Geometry check sheet. Reference: the model listing, model coordinates, mm. Face numbers are marked on the shaded views. A direction names the side the tool comes from. Round coordinates to 2 decimals unless told otherwise and drop trailing zeros. Write each loop counter-clockwise with the first axis right and the second up, starting at its lowest first coordinate (ties: lowest second). Pieces come first, ordered by that corner, then holes. Notation, with made-up numbers: (-37.75, 17) - (-32.75, 17) arc R16 ccw to (-32.75, 41) - close; hole circle Ø2 at (-12.5, -36.5). An arc over 180 degrees is marked (long way). Return JSON: item names as keys, results as strings. Group by question number.
from build123d import *

# Parameters (mm, degrees)
BOSS_EXTRU_1_DEPTH      = 1
ESQUISSE2_R             = 0.5
ENL_V_MAT_EXTRU_1_DEPTH = 10
ENL_V_MAT_EXTRU_2_DEPTH = 0.01
ENL_V_START             = -1
ENL_V_MAT_EXTRU_3_DEPTH = 0.01
BOSS_EXTRU_2_DEPTH      = 1.5
BOSS_EXTRU_2_DEPTH_BACK = 5.1
ESQUISSE5_R             = 2.275332805
BOSS_EXTRU_3_DEPTH      = 3.2
ENL_V_START_2           = -0.6
ESQUISSE6_R             = 2.275332805
ESQUISSE6_R_2           = 1.7
ENL_V_MAT_EXTRU_4_DEPTH = 2
ESQUISSE7_W             = 1.97090018
ESQUISSE7_H             = 3.898474417
ESQUISSE7_W_2           = 0.989857895
ESQUISSE7_H_2           = 1.612554693
ESQUISSE7_W_3           = 1.027355852
ESQUISSE7_W_4           = 1.146705559
ESQUISSE7_H_3           = 1.806710228
BOSS_EXTRU_4_DEPTH      = 1.5
ESQUISSE8_W             = 1.25807389
ESQUISSE8_H             = 0.666039119
ESQUISSE8_W_2           = 0.69364074
ESQUISSE8_H_2           = 1.255273727
BOSS_EXTRU_5_DEPTH      = 0.5
ESQUISSE9_W             = 3.84822602
ESQUISSE9_H             = 0.777045638
ENL_V_MAT_EXTRU_5_DEPTH = 1
CHANFREIN1_SIZE         = 0.4
ESQUISSE10_W            = 3.228737269
ESQUISSE10_H            = 1.612554693
ENL_V_MAT_EXTRU_6_DEPTH = 0.75
ESQUISSE11_W            = 1.213675147
ESQUISSE11_H            = 1.927537991
ENL_V_MAT_EXTRU_7_DEPTH = 0.5
ESQUISSE12_W            = 1.97090018
ESQUISSE12_H            = 3.898474417
BOSS_EXTRU_6_DEPTH      = 0.25
CHANFREIN2_SIZE         = 0.2
ENL_V_MAT_EXTRU_8_DEPTH = 6.25


with BuildPart() as part:
    # Esquisse1 → Boss.-Extru.1 (new body)
    with BuildSketch(Plane.XY):
        with BuildLine():
            Line((0, 11.3), (0.8, 12.1))
            Line((0.8, 12.1), (12.9, 12.1))
            ThreePointArc((12.9, 12.1), (13.5, 11.5), (14.1, 12.1))
            Line((14.1, 12.1), (15.2, 12.1))
            Line((15.2, 12.1), (16, 11.3))
            Line((16, 11.3), (16, 0.8))
            Line((16, 0.8), (15.2, 0))
            Line((15.2, 0), (14.1, 0))
            ThreePointArc((14.1, 0), (13.5, 0.6), (12.9, 0))
            Line((12.9, 0), (0.8, 0))
            Line((0.8, 0), (0, 0.8))
            Line((0, 0.8), (0, 11.3))
        make_face()
    extrude(amount=BOSS_EXTRU_1_DEPTH)

    # Esquisse2 → Enl_v. mat.-Extru.1 (cut)
    with BuildSketch(Plane.XY.offset(1)):
        with Locations((0.85, 10.25)):
            Circle(ESQUISSE2_R)
        with Locations((0.85, 1.85)):
            Circle(ESQUISSE2_R)
    extrude(amount=-ENL_V_MAT_EXTRU_1_DEPTH, mode=Mode.SUBTRACT)

    # Esquisse3 → Enl_v. mat.-Extru.2 (cut)
    with BuildSketch(Plane.XY.offset(1)):
        with BuildLine():
            Line((1.5, 9.2), (0.2, 9.2))
            ThreePointArc((0.2, 9.2), (0.058578644, 9.258578644), (0, 9.4))
            Line((0, 9.4), (0, 11.1))
            ThreePointArc((0, 11.1), (0.058578644, 11.241421356), (0.2, 11.3))
            Line((0.2, 11.3), (1.5, 11.3))
            ThreePointArc((1.5, 11.3), (1.641421356, 11.241421356), (1.7, 11.1))
            Line((1.7, 11.1), (1.7, 9.4))
            ThreePointArc((1.7, 9.4), (1.641421356, 9.258578644), (1.5, 9.2))
        make_face()
        with BuildLine():
            Line((1.5, 2.9), (0.2, 2.9))
            ThreePointArc((0.2, 2.9), (0.058578644, 2.841421356), (0, 2.7))
            Line((0, 2.7), (0, 1))
            ThreePointArc((0, 1), (0.058578644, 0.858578644), (0.2, 0.8))
            Line((0.2, 0.8), (1.5, 0.8))
            ThreePointArc((1.5, 0.8), (1.641421356, 0.858578644), (1.7, 1))
            Line((1.7, 1), (1.7, 2.7))
            ThreePointArc((1.7, 2.7), (1.641421356, 2.841421356), (1.5, 2.9))
        make_face()
    extrude(amount=-ENL_V_MAT_EXTRU_2_DEPTH, mode=Mode.SUBTRACT)

    # Esquisse3_2 → Enl_v. mat.-Extru.3 (cut)
    with BuildSketch(Plane.XY.offset(1).offset(ENL_V_START)):
        with BuildLine():
            Line((1.5, 9.2), (0.2, 9.2))
            ThreePointArc((0.2, 9.2), (0.058578644, 9.258578644), (0, 9.4))
            Line((0, 9.4), (0, 11.1))
            ThreePointArc((0, 11.1), (0.058578644, 11.241421356), (0.2, 11.3))
            Line((0.2, 11.3), (1.5, 11.3))
            ThreePointArc((1.5, 11.3), (1.641421356, 11.241421356), (1.7, 11.1))
            Line((1.7, 11.1), (1.7, 9.4))
            ThreePointArc((1.7, 9.4), (1.641421356, 9.258578644), (1.5, 9.2))
        make_face()
        with BuildLine():
            Line((1.5, 2.9), (0.2, 2.9))
            ThreePointArc((0.2, 2.9), (0.058578644, 2.841421356), (0, 2.7))
            Line((0, 2.7), (0, 1))
            ThreePointArc((0, 1), (0.058578644, 0.858578644), (0.2, 0.8))
            Line((0.2, 0.8), (1.5, 0.8))
            ThreePointArc((1.5, 0.8), (1.641421356, 0.858578644), (1.7, 1))
            Line((1.7, 1), (1.7, 2.7))
            ThreePointArc((1.7, 2.7), (1.641421356, 2.841421356), (1.5, 2.9))
        make_face()
    extrude(amount=ENL_V_MAT_EXTRU_3_DEPTH, mode=Mode.SUBTRACT)

    # Esquisse4 → Boss.-Extru.2 (add, two sides)
    with BuildSketch(Plane(origin=(16, 0, 0), x_dir=(0, 0, -1), z_dir=(1, 0, 0))) as boss_extru_2_sk:
        with BuildLine():
            Line((-4.2, 3.2), (-4.2, 8.9))
            ThreePointArc((-4.2, 8.9), (-2.6, 10.5), (-1, 8.9))
            Line((-1, 8.9), (-1, 3.2))
            ThreePointArc((-1, 3.2), (-2.6, 1.6), (-4.2, 3.2))
        make_face()
    extrude(amount=BOSS_EXTRU_2_DEPTH)
    extrude(boss_extru_2_sk.sketch, amount=-BOSS_EXTRU_2_DEPTH_BACK)

    # Esquisse5 → Boss.-Extru.3 (add)
    with BuildSketch(Plane.XY.offset(1)):
        with Locations((4.830231602, 2.627298973)):
            Circle(ESQUISSE5_R)
    extrude(amount=BOSS_EXTRU_3_DEPTH)

    # Esquisse6 → Enl_v. mat.-Extru.4 (cut)
    with BuildSketch(Plane.XY.offset(4.2).offset(ENL_V_START_2)):
        with Locations((4.830231602, 2.627298973)):
            Circle(ESQUISSE6_R)
        with Locations((4.830231602, 2.627298973)):
            Circle(ESQUISSE6_R_2, mode=Mode.SUBTRACT)
    extrude(amount=-ENL_V_MAT_EXTRU_4_DEPTH, mode=Mode.SUBTRACT)

    # Esquisse7 → Boss.-Extru.4 (add)
    with BuildSketch(Plane.XY.offset(1)):
        Polygon((4.12719031, 7.97411301), (4.460209869, 7.97411301), (4.460209869, 8.751158648), (5.200253335, 8.751158648), (5.200253335, 7.97411301), (5.644279414, 7.97411301), (5.644279414, 8.751158648), (6.310318533, 8.751158648), (6.310318533, 7.97411301), (6.754344612, 7.97411301), (6.754344612, 6.087002173), (6.310318533, 6.087002173), (6.310318533, 5.309956535), (5.644279414, 5.309956535), (5.644279414, 6.087002173), (5.200253335, 6.087002173), (5.200253335, 5.309956535), (4.460209869, 5.309956535), (4.460209869, 6.087002173), (4.12719031, 6.087002173), (4.12719031, 5.309956535), (3.387146845, 5.309956535), (3.387146845, 6.087002173), (2.906118592, 6.087002173), (2.906118592, 7.97411301), (3.387146845, 7.97411301), (3.387146845, 8.751158648), (4.12719031, 8.751158648), align=None)
        with Locations((8.659747019, 7.97411301)):
            Rectangle(ESQUISSE7_W, ESQUISSE7_H)
        with Locations((3.757168577, 10.711710291)):
            Rectangle(ESQUISSE7_W_2, ESQUISSE7_H_2)
        with Locations((5.977298973, 10.711710291)):
            Rectangle(ESQUISSE7_W_3, ESQUISSE7_H_2)
        with Locations((1.618258193, 6.024875801)):
            Rectangle(ESQUISSE7_W_4, ESQUISSE7_H_3)
    extrude(amount=BOSS_EXTRU_4_DEPTH)

    # Esquisse8 → Boss.-Extru.5 (add)
    with BuildSketch(Plane.XY.offset(1)):
        with Locations((8.548950015, 5.217451102)):
            Rectangle(ESQUISSE8_W, ESQUISSE8_H)
        with Locations((10.079839929, 3.846970609)):
            Rectangle(ESQUISSE8_W_2, ESQUISSE8_H_2)
    extrude(amount=BOSS_EXTRU_5_DEPTH)

    # Esquisse9 → Enl_v. mat.-Extru.5 (cut)
    with BuildSketch(Plane.XY.offset(2.5)):
        with Locations((4.830231602, 8.362635829)):
            Rectangle(ESQUISSE9_W, ESQUISSE9_H)
        with Locations((4.830231602, 5.698479354)):
            Rectangle(ESQUISSE9_W, ESQUISSE9_H)
    extrude(amount=-ENL_V_MAT_EXTRU_5_DEPTH, mode=Mode.SUBTRACT)

    # Chanfrein1
    chanfrein1_edges = [part.edges().sort_by_distance(p)[0] for p in [
        (3.757168577, 5.309956535, 1.5),
        (4.830231602, 5.309956535, 1.5),
        (5.977298973, 5.309956535, 1.5),
        (5.977298973, 8.751158648, 1.5),
        (4.830231602, 8.751158648, 1.5),
        (3.757168577, 8.751158648, 1.5),
    ]]
    chamfer(chanfrein1_edges, length=CHANFREIN1_SIZE)

    # Esquisse10 → Enl_v. mat.-Extru.6 (cut)
    with BuildSketch(Plane.XY.offset(2.5)):
        with Locations((4.876608265, 10.711710291)):
            Rectangle(ESQUISSE10_W, ESQUISSE10_H)
    extrude(amount=-ENL_V_MAT_EXTRU_6_DEPTH, mode=Mode.SUBTRACT)

    # Esquisse11 → Enl_v. mat.-Extru.7 (cut)
    with BuildSketch(Plane.XY.offset(2.5)):
        with Locations((1.651742986, 6.085289683)):
            Rectangle(ESQUISSE11_W, ESQUISSE11_H)
    extrude(amount=-ENL_V_MAT_EXTRU_7_DEPTH, mode=Mode.SUBTRACT)

    # Esquisse12 → Boss.-Extru.6 (add)
    with BuildSketch(Plane.XY.offset(2.5)):
        with Locations((8.659747019, 7.97411301)):
            Rectangle(ESQUISSE12_W, ESQUISSE12_H)
    extrude(amount=BOSS_EXTRU_6_DEPTH)

    # Chanfrein2
    chanfrein2_edges = [part.edges().sort_by_distance(p)[0] for p in [
        (4.252097525, 10.71171029, 1.75),
        (5.463621047, 10.71171029, 1.75),
        (3.757168577, 9.905432944, 1.75),
        (5.977298973, 9.905432944, 1.75),
        (3.757168577, 11.517987637, 1.75),
        (5.977298973, 11.517987637, 1.75),
        (6.490976899, 10.71171029, 1.75),
        (3.26223963, 10.71171029, 1.75),
    ]]
    chamfer(chanfrein2_edges, length=CHANFREIN2_SIZE)

    # Esquisse13 → Enl_v. mat.-Extru.8 (cut)
    with BuildSketch(Plane(origin=(17.5, 0, 0), x_dir=(0, 0, -1), z_dir=(1, 0, 0))):
        with BuildLine():
            Line((-1.2, 3.2), (-1.2, 8.9))
            ThreePointArc((-1.2, 8.9), (-2.6, 10.3), (-4, 8.9))
            Line((-4, 8.9), (-4, 3.2))
            ThreePointArc((-4, 3.2), (-2.6, 1.8), (-1.2, 3.2))
        make_face()
        with BuildLine():
            Line((-2.2, 3.2), (-2.2, 8.9))
            ThreePointArc((-2.2, 8.9), (-2.6, 9.3), (-3, 8.9))
            Line((-3, 8.9), (-3, 3.2))
            ThreePointArc((-3, 3.2), (-2.6, 2.8), (-2.2, 3.2))
        make_face(mode=Mode.SUBTRACT)
    extrude(amount=-ENL_V_MAT_EXTRU_8_DEPTH, mode=Mode.SUBTRACT)


solid = part.part
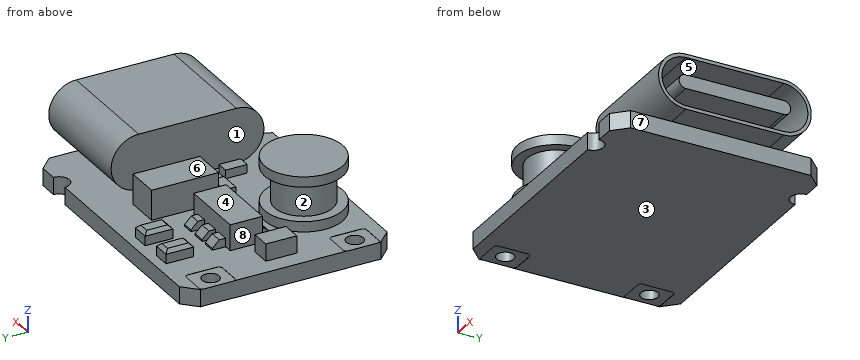
1. Section check C-C (x = 12.5). Enter the section's corners in (y, z), and give its area (3 significant figures).
2. Material ranges on line 1 along Y through (x, z) = (0.85, 0.75); line 2 along Z through (x, y) = (15.25, 5.75); line 3 along Z through (x, y) = (14.5, 2.5), recorded low to high.
3. Tool access check on the marked faces 1, 2, 3, 4 and 5. Record the directions out of +Z, -Z, +X, -X, +Y, -Y that give a thin tool (end or side, any length) a straight path to the whole face; none if there is none.
4. Section check A-A (x = 16.5). Enter the section's corners in (y, z), and give its area (3 significant figures).
5. Section check D-D (y = 7.25). Enter the section's corners in (x, z), and give its area (3 significant figures).
6. Section check B-B (z = 0.3). Enter the section's corners in (x, y).
7. Depth check by flat-ended pin: pin 1 Ø4.5 at (x, y) = (14, 5.5) entering from -Z; pin 2 Ø1 at (x, z) = (3.5, 2) entering from +Y; pin 3 Ø0.5 at (y, z) = (6, 1.5) entering from -X; pin 4 Ø0.6 at (x, y) = (2, 5.5) entering from +Z. Enter the tip coordinate at first touch or a pass-through.
8. Mould release check, pull along X, two halves, no side actions. Record for the marked faces 6, 7 and 8: pulls with the +X half, pulls with the -X half, needs draft (parallel to the pull), parting line crosses it, or undercut.
Result sheet:
{
 "1": {"outline": "(0, 0) - (12.1, 0) - (12.1, 1) - (8.9, 1) arc R1.6 ccw to (8.9, 4.2) - (3.2, 4.2) arc R1.6 ccw to (3.2, 1) - (0, 1) - close; (3.2, 2.2) - (8.9, 2.2) arc R0.4 ccw to (8.9, 3) - (3.2, 3) arc R0.4 ccw to start; hole (3.2, 1.2) - (8.9, 1.2) arc R1.4 ccw to (8.9, 4) - (3.2, 4) arc R1.4 ccw to start", "area": "21.3 mm²"},
 "2": {"line 1": "y = 0 to 1.35, 2.35 to 9.75, 10.75 to 12.1", "line 2": "z = 0 to 1.2, 2.2 to 3, 4 to 4.2", "line 3": "z = 0 to 1, 1.16 to 1.39, 3.81 to 4.04"},
 "3": {"face 1": "+Z, +Y, -Y", "face 2": "none", "face 3": "-Z, +X, -X, +Y, -Y", "face 4": "+Z, -X, +Y", "face 5": "+X"},
 "4": {"outline": "(3.2, 1) - (8.9, 1) arc R1.6 ccw to (8.9, 4.2) - (3.2, 4.2) arc R1.6 ccw to start; (3.2, 2.2) - (8.9, 2.2) arc R0.4 ccw to (8.9, 3) - (3.2, 3) arc R0.4 ccw to start; hole (3.2, 1.2) - (8.9, 1.2) arc R1.4 ccw to (8.9, 4) - (3.2, 4) arc R1.4 ccw to start", "area": "9.23 mm²"},
 "5": {"outline": "(0, 0) - (16, 0) - (16, 1) - (17.5, 1) - (17.5, 1.2) - (11.25, 1.2) - (11.25, 2.2) - (17.5, 2.2) - (17.5, 3) - (11.25, 3) - (11.25, 4) - (17.5, 4) - (17.5, 4.2) - (10.9, 4.2) - (10.9, 1) - (9.65, 1) - (9.65, 2.75) - (7.67, 2.75) - (7.67, 1) - (6.75, 1) - (6.75, 2.5) - (2.91, 2.5) - (2.91, 1) - (0, 1) - close", "area": "33.8 mm²"},
 "6": {"outline": "(0, 0.8) - (0.8, 0) - (12.9, 0) arc R0.6 cw to (14.1, 0) - (15.2, 0) - (16, 0.8) - (16, 11.3) - (15.2, 12.1) - (14.1, 12.1) arc R0.6 cw to (12.9, 12.1) - (0.8, 12.1) - (0, 11.3) - close; hole circle Ø1 at (0.85, 1.85); hole circle Ø1 at (0.85, 10.25)"},
 "7": {"pin 1": "stops at z = 0", "pin 2": "stops at y = 11.52", "pin 3": "stops at x = 1.04", "pin 4": "stops at z = 2"},
 "8": {"face 6": "needs draft", "face 7": "pulls with the +X half", "face 8": "undercut"}
}
